```python
from build123d import *

# Parameters (mm, degrees)
SKETCH1_W           = 32
SKETCH1_H           = 28
BOSS_EXTRUDE1_DEPTH = 1
SKETCH2_W           = 38
SKETCH2_H           = 34
SKETCH2_W_2         = 32
SKETCH2_H_2         = 28
BOSS_EXTRUDE2_DEPTH = 16
SKETCH3_W           = 31
SKETCH3_H           = 3
CUT_EXTRUDE1_DEPTH  = 16
SKETCH4_R           = 0.6
CUT_EXTRUDE2_DEPTH  = 61
BOSS_EXTRUDE3_REACH = 44.107
SKETCH9_R           = 0.6
CUT_EXTRUDE3_DEPTH  = 45
SKETCH10_W          = 20.681714782
SKETCH10_H          = 4.865607423
BOSS_EXTRUDE4_DEPTH = 3
SKETCH11_W          = 20.21758054
SKETCH11_H          = 4.689593046
BOSS_EXTRUDE5_DEPTH = 3
CUT_EXTRUDE5_DEPTH  = 43.107006543


with BuildPart() as part:
    # Sketch1 → Boss-Extrude1 (new body)
    with BuildSketch(Plane(origin=(0, 0, 0), x_dir=(1, 0, 0), z_dir=(0, 1, 0))):
        Rectangle(SKETCH1_W, SKETCH1_H)
    extrude(amount=BOSS_EXTRUDE1_DEPTH)

    # Sketch2 → Boss-Extrude2 (add)
    with BuildSketch(Plane(origin=(0, 0, 0), x_dir=(1, 0, 0), z_dir=(0, 1, 0))):
        Rectangle(SKETCH2_W, SKETCH2_H)
        Rectangle(SKETCH2_W_2, SKETCH2_H_2, mode=Mode.SUBTRACT)
    extrude(amount=BOSS_EXTRUDE2_DEPTH)

    # Sketch3 → Cut-Extrude1 (cut)
    with BuildSketch(Plane(origin=(0, 16, 0), x_dir=(1, 0, 0), z_dir=(0, 1, 0))):
        with Locations((-0.5, 15.5)):
            Rectangle(SKETCH3_W, SKETCH3_H)
        with Locations((-0.5, -15.5)):
            Rectangle(SKETCH3_W, SKETCH3_H)
    extrude(amount=-CUT_EXTRUDE1_DEPTH, mode=Mode.SUBTRACT)

    # Sketch4 → Cut-Extrude2 (cut)
    with BuildSketch(Plane(origin=(19, 0, 0), x_dir=(0, 0, -1), z_dir=(1, 0, 0))):
        with Locations((-7, 15)):
            Circle(SKETCH4_R)
        with Locations((-5.5, 15)):
            Circle(SKETCH4_R)
        with Locations((-4, 15)):
            Circle(SKETCH4_R)
        with Locations((-2.5, 15)):
            Circle(SKETCH4_R)
        with Locations((-1, 15)):
            Circle(SKETCH4_R)
        with Locations((0.5, 15)):
            Circle(SKETCH4_R)
        with Locations((2, 15)):
            Circle(SKETCH4_R)
        with Locations((3.5, 15)):
            Circle(SKETCH4_R)
        with Locations((5, 15)):
            Circle(SKETCH4_R)
        with Locations((6.5, 15)):
            Circle(SKETCH4_R)
        with Locations((-5.5, 10)):
            Circle(SKETCH4_R)
        with Locations((-4, 10)):
            Circle(SKETCH4_R)
        with Locations((-2.5, 10)):
            Circle(SKETCH4_R)
        with Locations((-1, 10)):
            Circle(SKETCH4_R)
        with Locations((0.5, 10)):
            Circle(SKETCH4_R)
        with Locations((2, 10)):
            Circle(SKETCH4_R)
        with Locations((3.5, 10)):
            Circle(SKETCH4_R)
        with Locations((5, 10)):
            Circle(SKETCH4_R)
        with Locations((6.5, 10)):
            Circle(SKETCH4_R)
        with Locations((-7, 10)):
            Circle(SKETCH4_R)
    extrude(amount=-CUT_EXTRUDE2_DEPTH, mode=Mode.SUBTRACT)

    # Boss-Extrude3: up to this face of the body (flat: up to its plane)
    boss_extrude3_end = Plane(part.part.faces().sort_by_distance((-17.5, 8, -17))[0])
    # Sketch6 → Boss-Extrude3 (add, up to the picked face)
    with BuildSketch(Plane.XY.offset(17), mode=Mode.PRIVATE) as boss_extrude3_sk1:
        Polygon((-16, 13.882344073), (-14.6, 12.018654658), (-16, 8.736052102), align=None)
    boss_extrude3_tool1 = split(extrude(boss_extrude3_sk1.sketch, amount=-BOSS_EXTRUDE3_REACH, mode=Mode.PRIVATE), bisect_by=boss_extrude3_end, keep=Keep.BOTH, mode=Mode.PRIVATE)
    # Sketch6 → Boss-Extrude3 (add, up to the picked face)
    with BuildSketch(Plane.XY.offset(17), mode=Mode.PRIVATE) as boss_extrude3_sk2:
        Polygon((14.6, 12.018654658), (16, 8.736052102), (16, 13.882344073), align=None)
    boss_extrude3_tool2 = split(extrude(boss_extrude3_sk2.sketch, amount=-BOSS_EXTRUDE3_REACH, mode=Mode.PRIVATE), bisect_by=boss_extrude3_end, keep=Keep.BOTH, mode=Mode.PRIVATE)
    add(boss_extrude3_tool1.solids().sort_by(Axis((-15.533333, 11.545684, 17), (0, 0, -1)))[0])
    add(boss_extrude3_tool2.solids().sort_by(Axis((15.533333, 11.545684, 17), (0, 0, -1)))[0])

    # Sketch9 → Cut-Extrude3 (cut)
    with BuildSketch(Plane.ZY.offset(19)):
        with Locations((-6.5, 5)):
            Circle(SKETCH9_R)
        with Locations((-5, 5)):
            Circle(SKETCH9_R)
        with Locations((-3.5, 5)):
            Circle(SKETCH9_R)
        with Locations((-2, 5)):
            Circle(SKETCH9_R)
        with Locations((-0.5, 5)):
            Circle(SKETCH9_R)
        with Locations((1, 5)):
            Circle(SKETCH9_R)
        with Locations((2.5, 5)):
            Circle(SKETCH9_R)
        with Locations((4, 5)):
            Circle(SKETCH9_R)
        with Locations((5.5, 5)):
            Circle(SKETCH9_R)
        with Locations((7, 5)):
            Circle(SKETCH9_R)
    extrude(amount=-CUT_EXTRUDE3_DEPTH, mode=Mode.SUBTRACT)

    # Sketch10 → Boss-Extrude4 (add)
    with BuildSketch(Plane.ZY.offset(19)):
        with Locations((1.876379269, 9.706359038)):
            Rectangle(SKETCH10_W, SKETCH10_H)
    extrude(amount=-BOSS_EXTRUDE4_DEPTH)

    # Sketch11 → Boss-Extrude5 (add)
    with BuildSketch(Plane(origin=(19, 0, 0), x_dir=(0, 0, -1), z_dir=(1, 0, 0))):
        with Locations((0.622743722, 10.359232414)):
            Rectangle(SKETCH11_W, SKETCH11_H)
    extrude(amount=-BOSS_EXTRUDE5_DEPTH)

    # Sketch12 → Cut-Extrude5 (cut, through all)
    with BuildSketch(Plane.XY.offset(17)):
        Polygon((14.6, 12.018654658), (16.041364921, 13.52892304), (16.041364921, 16), (15, 16), (13.555828546, 12.018654658), (11.7448085, 12.149887785), (9.441904284, 1.248003239), (15.747668413, 1.248003239), (15.747668413, 9.327698039), (14.882100771, 11.357208436), align=None)
    extrude(amount=-CUT_EXTRUDE5_DEPTH, mode=Mode.SUBTRACT)


solid = part.part
```
Geometry: final body of the model. Coordinates: model frame, mm. A direction names the side the tool comes from. Round coordinates to 2 decimals unless told otherwise and drop trailing zeros. Order: outer loops, then holes, each group sorted by start corner. A loop starts at its lowest first (then second) coordinate and runs counter-clockwise, first axis right, second up. Notation, with made-up numbers: (58, 1.5) -> (99, 1.5) arc R14 cw to (99, 11.5) -> close; hole circle Ø8 at (-9, 84.25). An arc over 180 degrees is marked (long way). Use one line per item in the form item = value. Start each with the question number.
1. Cut plane C-C (z = -15). Return the cut outline in (x, y).
2. Cut plane A-A (y = 3.5). Return the cut outline in (x, z), then the cut area to 3 significant figures.
3. Line query: probe 1 along Y at (x, z) = (-17.05, 2.5); probe 2 along X at (y, z) = (7.75, -6.5); probe 3 along X at (y, z) = (5.75, -15). Output: solid intervals per line, ascending.
4. Draft query along Z for faces 1 (the face through (-15.31, 12.964, 0.238)), 2 (the face through (17.541, 15.595, -1.922)). Return one class per face: pulls with the +Z half, pulls with the -Z half, needs draft (parallel to the pull), parting line crosses it, or undercut.
5. Reachability of faces 3 (the face through (16, 4, 0)), 4 (the face through (-17.479, 15.506, 0.677)), 5 (the face through (15, 1, 16)) from +Z, -Z, +X, -X, +Y, -Y: full face, straight path, thin tool, end or side. Return the list, or none.
6. Cut plane B-B (z = 4). Count the separate pieces of the cut face and the enclosed holes in it, then the cut area to 3 significant figures.
Solution:
q1.outline = (-19, 0) -> (-16, 0) -> (-16, 8.74) -> (-14.6, 12.02) -> (-16, 13.88) -> (-16, 16) -> (-19, 16) -> close; (14.6, 12.02) -> (15.75, 9.33) -> (15.75, 1.25) -> (15, 1.25) -> (15, 0) -> (19, 0) -> (19, 16) -> (16.04, 16) -> (16.04, 13.53) -> close
q2.outline = (-19, -17) -> (-16, -17) -> (-16, 17) -> (-19, 17) -> close; (15.75, -17) -> (19, -17) -> (19, 17) -> (15.75, 17) -> (15.75, 14) -> (16, 14) -> (16, -14) -> (15.75, -14) -> close
q2.area = 206 mm^2
q3.probe_1 = 0 to 4.4, 5.6 to 14.4, 15.6 to 16
q3.probe_2 = -19 to -16, 16 to 19
q3.probe_3 = -19 to -16, 15.75 to 19
q4.face_1 = needs draft
q4.face_2 = undercut
q5.face_3 = none
q5.face_4 = +X, -X
q5.face_5 = +Z, -Y
q6.separate_pieces = 5
q6.enclosed_holes = 0
q6.area = 120 mm^2
